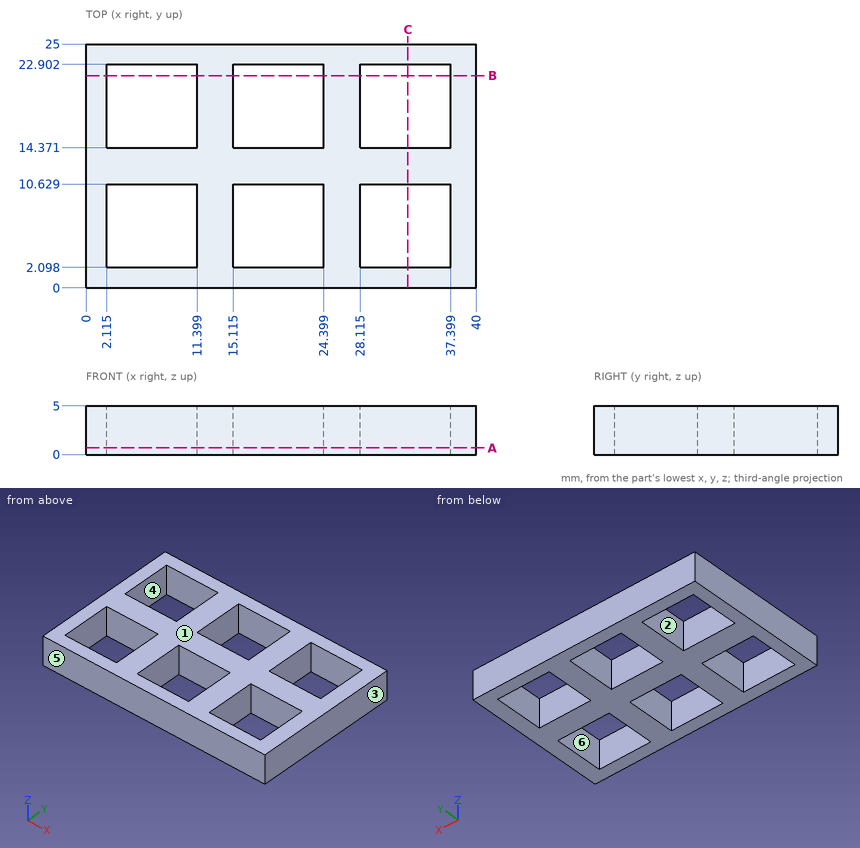
Geometry check sheet. Reference: drawing and pictorial views, mm from the part's lowest x, y, z. A direction names the side the tool comes from. Give positions to 0.01 mm unless a question says otherwise; leave off trailing zeros. Order: outer loops, then holes, each group sorted by start corner. A loop starts at its lowest first (then second) coordinate and runs counter-clockwise, first axis right, second up. Notation, with made-up numbers: (-28, 79) - (-15, 79) arc R21 cw to (-15, 111) - close; hole circle Ø8 at (-33.75, -34.5). An arc over 180 degrees is marked (long way). Answer as CSV lines item,"result".
1. Section check B-B (y = 21.75). Record the boundary of the cut face in (x, z) (1 decimal).
Result sheet:
outline,"(0, 0) - (2.1, 0) - (2.1, 5) - (0, 5) - close; (11.4, 0) - (15.1, 0) - (15.1, 5) - (11.4, 5) - close; (24.4, 0) - (28.1, 0) - (28.1, 5) - (24.4, 5) - close; (37.4, 0) - (40, 0) - (40, 5) - (37.4, 5) - close"
2. Go/stop test with a flat-tipped pin: P1, Ø1, axis at x = 34, y = 9.5, coming from the -Z side. Record where the tip stops, or that it passes through.
Result sheet:
P1,"through"
3. Section check C-C (x = 33). Record the boundary of the cut face in (y, z), then the cut area to 3 significant figures.
Result sheet:
outline,"(0, 0) - (2.1, 0) - (2.1, 5) - (0, 5) - close; (10.63, 0) - (14.37, 0) - (14.37, 5) - (10.63, 5) - close; (22.9, 0) - (25, 0) - (25, 5) - (22.9, 5) - close"
area,"39.7 mm²"
4. Mould release check, pull along X, two halves, no side actions. Record for the marked faces 1, 2, 3 and 4: released by +X, released by -X, zero draft, split by the parting line, or undercut.
Result sheet:
face 1,"zero draft"
face 2,"undercut"
face 3,"released by +X"
face 4,"undercut"
5. Tool access check on the marked faces 5 and 6. Record the directions out of +Z, -Z, +X, -X, +Y, -Y that give a thin tool (end or side, any length) a straight path to the whole face; none if there is none.
Result sheet:
face 5,"+Z, -Z, +X, -X, -Y"
face 6,"+Z, -Z"
6. Scan lines: probe 1 along Y at (x, z) = (18, 2.05); probe 2 along X at (y, z) = (17, 1.05) (1 decimal). Record each from-to range of solid material in increasing order. Write a range as from..to.
Result sheet:
probe 1,"0..2.1, 10.63..14.37, 22.9..25"
probe 2,"0..2.1, 11.4..15.1, 24.4..28.1, 37.4..40"
7. Section check A-A (z = 0.7). Record the boundary of the cut face in (x, y) (1 decimal).
Result sheet:
outline,"(0, 0) - (40, 0) - (40, 25) - (0, 25) - close; hole (2.1, 2.1) - (11.4, 2.1) - (11.4, 10.6) - (2.1, 10.6) - close; hole (2.1, 14.4) - (11.4, 14.4) - (11.4, 22.9) - (2.1, 22.9) - close; hole (15.1, 2.1) - (24.4, 2.1) - (24.4, 10.6) - (15.1, 10.6) - close; hole (15.1, 14.4) - (24.4, 14.4) - (24.4, 22.9) - (15.1, 22.9) - close; hole (28.1, 2.1) - (37.4, 2.1) - (37.4, 10.6) - (28.1, 10.6) - close; hole (28.1, 14.4) - (37.4, 14.4) - (37.4, 22.9) - (28.1, 22.9) - close"
